Work out the finished part from the listing and answer in its coordinate system (mm). A direction names the side the tool comes from. Give positions to 0.01 mm unless a question says otherwise; leave off trailing zeros. Write each loop counter-clockwise with the first axis right and the second up, starting at its lowest first coordinate (ties: lowest second). Pieces come first, ordered by that corner, then holes. Notation, with made-up numbers: (11, 31) -> (15, 31) arc R30 cw to (15, 59) -> close; hole circle Ø1 at (57.25, 36.25). An arc over 180 degrees is marked (long way). Write item = value, one per line. Start each with the question number.
from build123d import *

# Parameters (mm, degrees)
BOSS_EXTRUDE2_DEPTH = 5
SKETCH3_W           = 3
SKETCH3_H           = 94
SKETCH3_W_2         = 75
SKETCH3_H_2         = 31
BOSS_EXTRUDE4_DEPTH = 3
BOSS_EXTRUDE5_DEPTH = 3
SKETCH5_R           = 2
CUT_EXTRUDE1_DEPTH  = 5
SKETCH6_R           = 2
CUT_EXTRUDE2_DEPTH  = 3
SKETCH7_R           = 2
CUT_EXTRUDE3_DEPTH  = 8
FILLET1_R           = 5
FILLET2_R           = 5


with BuildPart() as part:
    # Sketch1 → Boss-Extrude2 (new body)
    with BuildSketch(Plane(origin=(0, 0, 0), x_dir=(1, 0, 0), z_dir=(0, 1, 0))):
        Polygon((-51.065846009, -44.178571429), (-59.065846009, -44.178571429), (-59.065846009, 49.821428571), (-51.065846009, 49.821428571), (-43.065846009, 49.821428571), (-43.065846009, 39.321428571), (-43.065846009, 34.321428571), (-38.065846009, 34.321428571), (26.934153991, 34.321428571), (31.934153991, 34.321428571), (31.934153991, 39.321428571), (31.934153991, 49.821428571), (39.934153991, 49.821428571), (47.934153991, 49.821428571), (47.934153991, -44.178571429), (39.934153991, -44.178571429), (31.934153991, -44.178571429), (31.934153991, -33.678571429), (31.934153991, -28.678571429), (26.934153991, -28.678571429), (-38.065846009, -28.678571429), (-43.065846009, -28.678571429), (-43.065846009, -33.678571429), (-43.065846009, -44.178571429), align=None)
        Polygon((-43.065846009, 13.321428571), (-43.065846009, -7.678571429), (-43.065846009, -12.678571429), (-38.065846009, -12.678571429), (26.934153991, -12.678571429), (31.934153991, -12.678571429), (31.934153991, -7.678571429), (31.934153991, 13.321428571), (31.934153991, 18.321428571), (26.934153991, 18.321428571), (-38.065846009, 18.321428571), (-43.065846009, 18.321428571), align=None, mode=Mode.SUBTRACT)
    extrude(amount=BOSS_EXTRUDE2_DEPTH)

    # Sketch3 → Boss-Extrude4 (add)
    # profile 1 of 5: a face of its own
    with BuildSketch(Plane(origin=(0, 5, 0), x_dir=(1, 0, 0), z_dir=(0, 1, 0))):
        with Locations((-57.565846009, 2.821428571)):
            Rectangle(SKETCH3_W, SKETCH3_H)
    # profile 2 of 5: a face of its own
    with BuildSketch(Plane(origin=(0, 5, 0), x_dir=(1, 0, 0), z_dir=(0, 1, 0))):
        with Locations((46.434153991, 2.821428571)):
            Rectangle(SKETCH3_W, SKETCH3_H)
    # profile 3 of 5: a face of its own
    with BuildSketch(Plane(origin=(0, 5, 0), x_dir=(1, 0, 0), z_dir=(0, 1, 0))):
        Polygon((-43.065846009, 49.821428571), (-46.065846009, 49.821428571), (-46.065846009, 34.321428571), (-46.065846009, 31.321428571), (31.934153991, 31.321428571), (34.934153991, 31.321428571), (34.934153991, 49.821428571), (31.934153991, 49.821428571), (31.934153991, 34.321428571), (-43.065846009, 34.321428571), align=None)
    # profile 4 of 5: a face of its own
    with BuildSketch(Plane(origin=(0, 5, 0), x_dir=(1, 0, 0), z_dir=(0, 1, 0))):
        Polygon((34.934153991, 21.321428571), (34.934153991, -12.678571429), (34.934153991, -15.678571429), (-46.065846009, -15.678571429), (-46.065846009, 21.321428571), (31.934153991, 21.321428571), align=None)
        with Locations((-5.565846009, 2.821428571)):
            Rectangle(SKETCH3_W_2, SKETCH3_H_2, mode=Mode.SUBTRACT)
    # profile 5 of 5: a face of its own
    with BuildSketch(Plane(origin=(0, 5, 0), x_dir=(1, 0, 0), z_dir=(0, 1, 0))):
        Polygon((-46.065846009, -44.178571429), (-43.065846009, -44.178571429), (-43.065846009, -28.678571429), (31.934153991, -28.678571429), (31.934153991, -44.178571429), (34.934153991, -44.178571429), (34.934153991, -28.678571429), (34.934153991, -25.678571429), (-46.065846009, -25.678571429), align=None)
    extrude(amount=BOSS_EXTRUDE4_DEPTH)

    # Sketch4 → Boss-Extrude5 (add)
    with BuildSketch(Plane(origin=(0, 5, 0), x_dir=(1, 0, 0), z_dir=(0, 1, 0))):
        Polygon((-46.065846009, -59.178571429), (-46.065846009, -29.178571429), (-56.065846009, -29.178571429), (-56.065846009, -59.178571429), (-51.065846009, -59.178571429), align=None)
        Polygon((39.934153991, -59.178571429), (44.934153991, -59.178571429), (44.934153991, -29.178571429), (34.934153991, -29.178571429), (34.934153991, -59.178571429), align=None)
        Polygon((-46.065846009, 34.821428571), (-46.065846009, 64.821428571), (-56.065846009, 64.821428571), (-56.065846009, 34.821428571), (-51.065846009, 34.821428571), align=None)
        Polygon((44.934153991, 34.821428571), (44.934153991, 64.821428571), (34.934153991, 64.821428571), (34.934153991, 34.821428571), (39.934153991, 34.821428571), align=None)
    extrude(amount=BOSS_EXTRUDE5_DEPTH)

    # Sketch5 → Cut-Extrude1 (cut)
    with BuildSketch(Plane(origin=(0, 5, 0), x_dir=(1, 0, 0), z_dir=(0, 1, 0))):
        with Locations(Location((-51.065846009, 26.321428571, 0), (0, 0, 270))):
            Circle(SKETCH5_R)
        with Locations(Location((39.934153991, 26.321428571, 0), (0, 0, 270))):
            Circle(SKETCH5_R)
        with Locations(Location((39.934153991, -20.678571429, 0), (0, 0, 270))):
            Circle(SKETCH5_R)
        with Locations(Location((-51.065846009, -20.678571429, 0), (0, 0, 270))):
            Circle(SKETCH5_R)
        with Locations(Location((-51.065846009, 2.821428571, 0), (0, 0, 270))):
            Circle(SKETCH5_R)
        with Locations(Location((39.934153991, 2.821428571, 0), (0, 0, 270))):
            Circle(SKETCH5_R)
        with Locations(Location((-51.065846009, 14.571428571, 0), (0, 0, 270))):
            Circle(SKETCH5_R)
        with Locations(Location((-51.065846009, -8.928571429, 0), (0, 0, 270))):
            Circle(SKETCH5_R)
        with Locations(Location((-5.565846009, 26.321428571, 0), (0, 0, 270))):
            Circle(SKETCH5_R)
        with Locations(Location((14.434153991, 26.321428571, 0), (0, 0, 270))):
            Circle(SKETCH5_R)
        with Locations(Location((24.434153991, 26.321428571, 0), (0, 0, 270))):
            Circle(SKETCH5_R)
        with Locations(Location((-25.565846009, 26.321428571, 0), (0, 0, 270))):
            Circle(SKETCH5_R)
        with Locations(Location((4.434153991, 26.321428571, 0), (0, 0, 270))):
            Circle(SKETCH5_R)
        with Locations(Location((-35.565846009, 26.321428571, 0), (0, 0, 270))):
            Circle(SKETCH5_R)
        with Locations(Location((-15.565846009, 26.321428571, 0), (0, 0, 270))):
            Circle(SKETCH5_R)
        with Locations(Location((-5.565846009, -20.678571429, 0), (0, 0, 270))):
            Circle(SKETCH5_R)
        with Locations(Location((14.434153991, -20.678571429, 0), (0, 0, 270))):
            Circle(SKETCH5_R)
        with Locations(Location((24.434153991, -20.678571429, 0), (0, 0, 270))):
            Circle(SKETCH5_R)
        with Locations(Location((-25.565846009, -20.678571429, 0), (0, 0, 270))):
            Circle(SKETCH5_R)
        with Locations(Location((4.434153991, -20.678571429, 0), (0, 0, 270))):
            Circle(SKETCH5_R)
        with Locations(Location((-35.565846009, -20.678571429, 0), (0, 0, 270))):
            Circle(SKETCH5_R)
        with Locations(Location((-15.565846009, -20.678571429, 0), (0, 0, 270))):
            Circle(SKETCH5_R)
        with Locations(Location((39.934153991, 14.571428571, 0), (0, 0, 270))):
            Circle(SKETCH5_R)
        with Locations(Location((39.934153991, -8.928571429, 0), (0, 0, 270))):
            Circle(SKETCH5_R)
    extrude(amount=-CUT_EXTRUDE1_DEPTH, mode=Mode.SUBTRACT)

    # Sketch6 → Cut-Extrude2 (cut)
    with BuildSketch(Plane.XZ.offset(-5)):
        with Locations(Location((39.934153991, -54.821428571, 0), (0, 0, 270))):
            Circle(SKETCH6_R)
        with Locations(Location((-51.065846009, -54.821428571, 0), (0, 0, 270))):
            Circle(SKETCH6_R)
        with Locations(Location((-51.065846009, 49.178571429, 0), (0, 0, 270))):
            Circle(SKETCH6_R)
        with Locations(Location((39.934153991, 49.178571429, 0), (0, 0, 270))):
            Circle(SKETCH6_R)
    extrude(amount=-CUT_EXTRUDE2_DEPTH, mode=Mode.SUBTRACT)

    # Sketch7 → Cut-Extrude3 (cut)
    with BuildSketch(Plane(origin=(0, 8, 0), x_dir=(1, 0, 0), z_dir=(0, 1, 0))):
        with Locations(Location((-51.065846009, 42.321428571, 0), (0, 0, 270))):
            Circle(SKETCH7_R)
        with Locations(Location((39.934153991, 42.321428571, 0), (0, 0, 270))):
            Circle(SKETCH7_R)
        with Locations(Location((-51.065846009, -36.678571429, 0), (0, 0, 270))):
            Circle(SKETCH7_R)
        with Locations(Location((39.934153991, -36.678571429, 0), (0, 0, 270))):
            Circle(SKETCH7_R)
    extrude(amount=-CUT_EXTRUDE3_DEPTH, mode=Mode.SUBTRACT)

    # Fillet1
    fillet1_edges = [part.edges().sort_by_distance(p)[0] for p in [
        (31.934153991, 4, 28.678571429),
        (-43.065846009, 4, 28.678571429),
        (-43.065846009, 4, -34.321428571),
        (31.934153991, 4, -34.321428571),
        (-43.065846009, 4, -18.321428571),
        (-43.065846009, 4, 12.678571429),
        (31.934153991, 4, 12.678571429),
        (31.934153991, 4, -18.321428571),
    ]]
    fillet(fillet1_edges, radius=FILLET1_R)

    # Fillet2
    # the kernel refuses this fillet: 5 mm, written as the material it takes off along each edge
    with BuildSketch(Plane(origin=(-46.065846009, 5, -31.321428571), x_dir=(1, 0, 0), z_dir=(0, 1, 0))) as fillet2_piece_1:
        with BuildLine():
            CenterArc((4.769696007, 5), FILLET2_R, 197.457603124, 72.542396876)
            Line((0, 3.5), (0, 0))
            Line((0, 0), (4.769696007, 0))
        make_face()
    extrude(amount=14.924240018, mode=Mode.SUBTRACT)
    with BuildSketch(Plane(origin=(34.934153991, 5, -31.321428571), x_dir=(0, 0, -1), z_dir=(0, 1, 0))) as fillet2_piece_2:
        with BuildLine():
            CenterArc((5, 4.769696007), FILLET2_R, 180, 72.542396876)
            Line((0, 4.769696007), (0, 0))
            Line((0, 0), (3.5, 0))
        make_face()
    extrude(amount=14.924240018, mode=Mode.SUBTRACT)
    with BuildSketch(Plane(origin=(-46.065846009, 5, 25.678571429), x_dir=(1, 0, 0), z_dir=(0, 1, 0))) as fillet2_piece_3:
        with BuildLine():
            CenterArc((4.769696007, -5), FILLET2_R, 90, 72.542396876)
            Line((0, -3.5), (0, 0))
            Line((0, 0), (4.769696007, 0))
        make_face()
    extrude(amount=14.924240018, mode=Mode.SUBTRACT)
    with BuildSketch(Plane(origin=(34.934153991, 5, 25.678571429), x_dir=(0, 0, 1), z_dir=(0, 1, 0))) as fillet2_piece_4:
        with BuildLine():
            CenterArc((5, -4.769696007), FILLET2_R, 107.457603124, 72.542396876)
            Line((0, -4.769696007), (0, 0))
            Line((0, 0), (3.5, 0))
        make_face()
    extrude(amount=14.924240018, mode=Mode.SUBTRACT)
    with BuildSketch(Plane(origin=(-46.065846009, 5, -21.321428571), x_dir=(0, 0, 1), z_dir=(0, 1, 0)), Plane(origin=(-46.065846009, 5, 15.678571429), x_dir=(1, 0, 0), z_dir=(0, 1, 0))) as fillet2_piece_5:
        with BuildLine():
            CenterArc((FILLET2_R, FILLET2_R), FILLET2_R, 180, 90)
            Line((0, FILLET2_R), (0, 0))
            Line((0, 0), (FILLET2_R, 0))
        make_face()
    extrude(amount=15.5, mode=Mode.SUBTRACT)
    with BuildSketch(Plane(origin=(34.934153991, 5, 15.678571429), x_dir=(-1, 0, 0), z_dir=(0, 1, 0)), Plane(origin=(34.934153991, 5, -21.321428571), x_dir=(0, 0, 1), z_dir=(0, 1, 0))) as fillet2_piece_6:
        with BuildLine():
            CenterArc((FILLET2_R, -FILLET2_R), FILLET2_R, 90, 90)
            Line((0, -FILLET2_R), (0, 0))
            Line((0, 0), (FILLET2_R, 0))
        make_face()
    extrude(amount=15.5, mode=Mode.SUBTRACT)


solid = part.part
(1) For faces 1 (the cylindrical face through (30.508, 3.944, 11.175)), 2 (the cylindrical face through (-41.64, 4.06, 30.18)), 3 (the cylindrical face through (33.087, 6.479, -32.264)), 4 (the flat face through (-51, 6, -64.821)), 5 (the flat face through (-43.066, 4, -44)), determine the directions among +Z, -Z, +X, -X, +Y, -Y from which every point of the face is accessible in a straight line to the end or side of a thin tool.
(2) Determine the mould class of faces 6 (the flat face through (-2, 8, 14)), 7 (the cylindrical face through (41.286, 2.535, 19.204)) for opening direction X: pulls with the +X half, pulls with the -X half, needs draft (parallel to the pull), parting line crosses it, or undercut.
(3) A cutting plane is placed at C-C, the plane z = -30. Write down the section's boundary in (x, y).
(4) A cutting plane is placed at D-D, the plane y = 6.25. State how many separate pieces and enclosed holes the cut face has, then the cut area to 3 significant figures.
(5) A cutting plane is placed at A-A, the plane z = -7. Write down the section's boundary in (x, y).
(6) A cutting plane is placed at B-B, the plane x = 0. Write down the section's boundary in (y, z), then the cut area to 3 significant figures.
(7) Find the intervals of material crossed by line 1 along Z through (x, y) = (2.5, 5.5); line 2 along Z through (x, y) = (-14, 0.5); line 3 along Z through (x, y) = (-32.5, 2), in increasing order.
(8) Each of these flat-tipped pins is pushed along its axis until it touches: pin 1 (10 mm diameter, centred on x = -33.5, z = -35, fed in from +Y); pin 2 (4.5 mm diameter, centred on x = -51.07, z = 8.93, fed in from +Y); pin 3 (1.5 mm diameter, centred on y = 7, z = -53.5, fed in from -X); pin 4 (0.9 mm diameter, centred on y = 6, z = 52, fed in from +X). Where does it stop, or does it pass through?
Results list:
q1.face_1 = +Y, -Y
q1.face_2 = +Z, +Y, -Y
q1.face_3 = +Y
q1.face_4 = -Z, +X, -X, +Y, -Y
q1.face_5 = -Z, +Y, -Y
q2.face_6 = needs draft
q2.face_7 = undercut
q3.outline = (-59.07, 0) -> (47.93, 0) -> (47.93, 8) -> (44.93, 8) -> (44.93, 5) -> (-56.07, 5) -> (-56.07, 8) -> (-59.07, 8) -> close
q4.separate_pieces = 2
q4.enclosed_holes = 10
q4.area = 3,010 mm²
q5.outline = (-59.07, 0) -> (-43.07, 0) -> (-43.07, 8) -> (-46.07, 8) -> (-46.07, 5) -> (-56.07, 5) -> (-56.07, 8) -> (-59.07, 8) -> close; (31.93, 0) -> (47.93, 0) -> (47.93, 8) -> (44.93, 8) -> (44.93, 5) -> (34.93, 5) -> (34.93, 8) -> (31.93, 8) -> close
q6.outline = (0, -34.32) -> (8, -34.32) -> (8, -31.32) -> (5, -31.32) -> (5, -21.32) -> (8, -21.32) -> (8, -18.32) -> (0, -18.32) -> close; (0, 12.68) -> (8, 12.68) -> (8, 15.68) -> (5, 15.68) -> (5, 25.68) -> (8, 25.68) -> (8, 28.68) -> (0, 28.68) -> close
q6.area = 196 mm²
q7.line_1 = -34.32 to -31.32, -21.32 to -18.32, 12.68 to 15.68, 25.68 to 28.68
q7.line_2 = -34.32 to -27.57, -25.08 to -18.32, 12.68 to 19.43, 21.92 to 28.68
q7.line_3 = -34.32 to -18.32, 12.68 to 28.68
q8.pin_1 = 8
q8.pin_2 = 5
q8.pin_3 = -56.07
q8.pin_4 = 44.93
